```python
from build123d import *

# Parameters (mm, degrees)
F0_R     = 3
F0_R_2   = 6.530293
F1_DEPTH = 25


with BuildPart() as f1:
    # F0 (on Front) → F1 (new body)
    with BuildSketch(Plane.XZ):
        with BuildLine():
            ThreePointArc((24.831743, -2.895608), (24.9579, -1.450246), (25, 0))
            ThreePointArc((25, 0), (24.95158, 1.555208), (24.806506, 3.104392))
            ThreePointArc((24.806506, 3.104392), (24.498901, 4.980347), (24.04964, 6.827504))
            ThreePointArc((24.04964, 6.827504), (23.056544, 9.664149), (21.730224, 12.361123))
            ThreePointArc((21.730224, 12.361123), (20.728137, 13.976564), (19.606198, 15.51119))
            ThreePointArc((19.606198, 15.51119), (17.603159, 17.751867), (15.345712, 19.735986))
            ThreePointArc((15.345712, 19.735986), (13.801702, 20.844976), (12.177889, 21.833438))
            ThreePointArc((12.177889, 21.833438), (9.469853, 23.137024), (6.624954, 24.106223))
            ThreePointArc((6.624954, 24.106223), (4.774083, 24.539929), (2.895608, 24.831743))
            ThreePointArc((2.895608, 24.831743), (-0.105152, 24.999779), (-3.104392, 24.806506))
            ThreePointArc((-3.104392, 24.806506), (-4.980347, 24.498901), (-6.827504, 24.04964))
            ThreePointArc((-6.827504, 24.04964), (-9.664149, 23.056544), (-12.361123, 21.730224))
            ThreePointArc((-12.361123, 21.730224), (-13.976564, 20.728137), (-15.51119, 19.606198))
            ThreePointArc((-15.51119, 19.606198), (-17.751867, 17.603159), (-19.735986, 15.345712))
            ThreePointArc((-19.735986, 15.345712), (-20.844976, 13.801702), (-21.833438, 12.177889))
            ThreePointArc((-21.833438, 12.177889), (-23.137024, 9.469853), (-24.106223, 6.624954))
            ThreePointArc((-24.106223, 6.624954), (-24.539929, 4.774083), (-24.831743, 2.895608))
            ThreePointArc((-24.831743, 2.895608), (-24.999779, -0.105152), (-24.806506, -3.104392))
            ThreePointArc((-24.806506, -3.104392), (-24.498901, -4.980347), (-24.04964, -6.827504))
            ThreePointArc((-24.04964, -6.827504), (-23.056544, -9.664149), (-21.730224, -12.361123))
            ThreePointArc((-21.730224, -12.361123), (-20.728137, -13.976564), (-19.606198, -15.51119))
            ThreePointArc((-19.606198, -15.51119), (-17.603159, -17.751867), (-15.345712, -19.735986))
            ThreePointArc((-15.345712, -19.735986), (-13.801702, -20.844976), (-12.177889, -21.833438))
            ThreePointArc((-12.177889, -21.833438), (-9.469853, -23.137024), (-6.624954, -24.106223))
            ThreePointArc((-6.624954, -24.106223), (-4.774083, -24.539929), (-2.895608, -24.831743))
            ThreePointArc((-2.895608, -24.831743), (0.105152, -24.999779), (3.104392, -24.806506))
            ThreePointArc((3.104392, -24.806506), (4.980347, -24.498901), (6.827504, -24.04964))
            ThreePointArc((6.827504, -24.04964), (9.664149, -23.056544), (12.361123, -21.730224))
            ThreePointArc((12.361123, -21.730224), (13.976564, -20.728137), (15.51119, -19.606198))
            ThreePointArc((15.51119, -19.606198), (17.751867, -17.603159), (19.735986, -15.345712))
            ThreePointArc((19.735986, -15.345712), (20.844976, -13.801702), (21.833438, -12.177889))
            ThreePointArc((21.833438, -12.177889), (23.137024, -9.469853), (24.106223, -6.624954))
            ThreePointArc((24.106223, -6.624954), (24.539929, -4.774083), (24.831743, -2.895608))
        make_face()
        with Locations((-5.740251, -13.858193)):
            Circle(F0_R, mode=Mode.SUBTRACT)
        with Locations((10.606602, -10.606602)):
            Circle(F0_R, mode=Mode.SUBTRACT)
        with Locations((-15, 0)):
            Circle(F0_R, mode=Mode.SUBTRACT)
        Circle(F0_R_2, mode=Mode.SUBTRACT)
        with Locations((13.858193, 5.740251)):
            Circle(F0_R, mode=Mode.SUBTRACT)
        with Locations((0, 15)):
            Circle(F0_R, mode=Mode.SUBTRACT)
        with BuildLine():
            ThreePointArc((24.806506, 3.104392), (24.95158, 1.555208), (25, 0))
            ThreePointArc((25, 0), (24.9579, -1.450246), (24.831743, -2.895608))
            Line((24.831743, -2.895608), (30.030659, -1.999731))
            Line((30.030659, -1.999731), (29.965095, 1.999731))
            Line((29.965095, 1.999731), (24.806506, 3.104392))
        make_face()
        with BuildLine():
            ThreePointArc((21.730224, 12.361123), (23.056544, 9.664149), (24.04964, 6.827504))
            Line((24.04964, 6.827504), (28.509975, 9.644725))
            Line((28.509975, 9.644725), (26.918874, 13.314656))
            Line((26.918874, 13.314656), (21.730224, 12.361123))
        make_face()
        with BuildLine():
            Line((28.449402, -9.619635), (24.106223, -6.624954))
            ThreePointArc((24.106223, -6.624954), (23.137024, -9.469853), (21.833438, -12.177889))
            Line((21.833438, -12.177889), (26.979447, -13.339746))
            Line((26.979447, -13.339746), (28.449402, -9.619635))
        make_face()
        with BuildLine():
            ThreePointArc((15.345712, 19.735986), (17.603159, 17.751867), (19.606198, 15.51119))
            Line((19.606198, 15.51119), (22.648906, 19.820859))
            Line((22.648906, 19.820859), (19.774499, 22.602546))
            Line((19.774499, 22.602546), (15.345712, 19.735986))
        make_face()
        with BuildLine():
            Line((22.602546, -19.774499), (19.735986, -15.345712))
            ThreePointArc((19.735986, -15.345712), (17.751867, -17.603159), (15.51119, -19.606198))
            Line((15.51119, -19.606198), (19.820859, -22.648906))
            Line((19.820859, -22.648906), (22.602546, -19.774499))
        make_face()
        with BuildLine():
            ThreePointArc((6.624954, 24.106223), (9.469853, 23.137024), (12.177889, 21.833438))
            Line((12.177889, 21.833438), (13.339746, 26.979447))
            Line((13.339746, 26.979447), (9.619635, 28.449402))
            Line((9.619635, 28.449402), (6.624954, 24.106223))
        make_face()
        with BuildLine():
            Line((13.314656, -26.918874), (12.361123, -21.730224))
            ThreePointArc((12.361123, -21.730224), (9.664149, -23.056544), (6.827504, -24.04964))
            Line((6.827504, -24.04964), (9.644725, -28.509975))
            Line((9.644725, -28.509975), (13.314656, -26.918874))
        make_face()
        with BuildLine():
            ThreePointArc((-3.104392, 24.806506), (-0.105152, 24.999779), (2.895608, 24.831743))
            Line((2.895608, 24.831743), (1.999731, 30.030659))
            Line((1.999731, 30.030659), (-1.999731, 29.965095))
            Line((-1.999731, 29.965095), (-3.104392, 24.806506))
        make_face()
        with BuildLine():
            Line((1.999731, -29.965095), (3.104392, -24.806506))
            ThreePointArc((3.104392, -24.806506), (0.105152, -24.999779), (-2.895608, -24.831743))
            Line((-2.895608, -24.831743), (-1.999731, -30.030659))
            Line((-1.999731, -30.030659), (1.999731, -29.965095))
        make_face()
        with BuildLine():
            ThreePointArc((-12.361123, 21.730224), (-9.664149, 23.056544), (-6.827504, 24.04964))
            Line((-6.827504, 24.04964), (-9.644725, 28.509975))
            Line((-9.644725, 28.509975), (-13.314656, 26.918874))
            Line((-13.314656, 26.918874), (-12.361123, 21.730224))
        make_face()
        with BuildLine():
            Line((-9.619635, -28.449402), (-6.624954, -24.106223))
            ThreePointArc((-6.624954, -24.106223), (-9.469853, -23.137024), (-12.177889, -21.833438))
            Line((-12.177889, -21.833438), (-13.339746, -26.979447))
            Line((-13.339746, -26.979447), (-9.619635, -28.449402))
        make_face()
        with BuildLine():
            ThreePointArc((-19.735986, 15.345712), (-17.751867, 17.603159), (-15.51119, 19.606198))
            Line((-15.51119, 19.606198), (-19.820859, 22.648906))
            Line((-19.820859, 22.648906), (-22.602546, 19.774499))
            Line((-22.602546, 19.774499), (-19.735986, 15.345712))
        make_face()
        with BuildLine():
            Line((-19.774499, -22.602546), (-15.345712, -19.735986))
            ThreePointArc((-15.345712, -19.735986), (-17.603159, -17.751867), (-19.606198, -15.51119))
            Line((-19.606198, -15.51119), (-22.648906, -19.820859))
            Line((-22.648906, -19.820859), (-19.774499, -22.602546))
        make_face()
        with BuildLine():
            ThreePointArc((-24.106223, 6.624954), (-23.137024, 9.469853), (-21.833438, 12.177889))
            Line((-21.833438, 12.177889), (-26.979447, 13.339746))
            Line((-26.979447, 13.339746), (-28.449402, 9.619635))
            Line((-28.449402, 9.619635), (-24.106223, 6.624954))
        make_face()
        with BuildLine():
            Line((-26.918874, -13.314656), (-21.730224, -12.361123))
            ThreePointArc((-21.730224, -12.361123), (-23.056544, -9.664149), (-24.04964, -6.827504))
            Line((-24.04964, -6.827504), (-28.509975, -9.644725))
            Line((-28.509975, -9.644725), (-26.918874, -13.314656))
        make_face()
        with BuildLine():
            ThreePointArc((-24.806506, -3.104392), (-24.999779, -0.105152), (-24.831743, 2.895608))
            Line((-24.831743, 2.895608), (-30.030659, 1.999731))
            Line((-30.030659, 1.999731), (-29.965095, -1.999731))
            Line((-29.965095, -1.999731), (-24.806506, -3.104392))
        make_face()
    extrude(amount=F1_DEPTH)


solid = f1.part
```
Can you work these out from the model? Positions are in its coordinate system, mm. A direction names the side the tool comes from. Give positions to 0.01 mm unless a question says otherwise; leave off trailing zeros. Order: outer loops, then holes, each group sorted by start corner. A loop starts at its lowest first (then second) coordinate and runs counter-clockwise, first axis right, second up. Notation, with made-up numbers: (-25.5, 4) - (-8.5, 4) arc R11 cw to (-8.5, 15) - close; hole circle Ø11 at (29, 55). An arc over 180 degrees is marked (long way). Use a Markdown table: item, result. Add a question column.
Q1. If we section it at B-B on x = 0: Write out the boundary of the cut face in (y, z), plus the area to 3 significant figures.
Q2. If we section it at D-D on y = -14: Count the separate pieces of the cut face and the enclosed holes in it, plus the area to 3 significant figures.
Q3. If we mould it in two halves opening along X, with no side actions, what happens to faces 1 (the flat face through (0, 0, 7)), 2 (the flat face through (-8.216, -12.325, 26.249)), 3 (the flat face through (-27.704, -12.325, 11.506))? For each: released by +X, released by -X, zero draft, split by the parting line, or undercut.
Q4. I'm going to push flat-ended pins straight in: pin 1 (2 mm diameter, centred on y = -20.5, z = 15.5, fed in from -X); pin 2 (1.5 mm diameter, centred on x = -10.5, y = -21.5, fed in from +Z); pin 3 (10 mm diameter, centred on x = 8.5, y = -10, fed in from -Z). Where does each tip first touch, or does it pass through?
Q5. If we section it at A-A on x = -17: Write out the boundary of the cut face in (y, z), plus the area to 3 significant figures.
Q6. If we section it at C-C on z = 0: Write out the boundary of the cut face in (x, y).
Q7. Please list where these lines run through material, in increasing order: line 1 along Z through (x, y) = (22, -5); line 2 along X through (y, z) = (-4.75, -25.5); line 3 along X through (y, z) = (-16.5, -25).
Q8. On a 3-axis mill with a long thin cutter (end or side, diameter ignored), from which of +Z, -Z, +X, -X, +Y, -Y can I reach the whole of each face in a straight line? I mean faces 4 (the flat face through (-21.232, -12.325, -21.192)), 5 (the flat face through (2.454, -12.325, 27.395)), 6 (the flat face through (2.544, -12.325, -27.422)), 7 (the cylindrical face through (-20.83, -12.325, 13.824)). Say none if no direction works.
Answers follow:
| question | item | result |
|---|---|---|
| 1 | outline | (-25, -30) - (0, -30) - (0, -6.53) - (-25, -6.53) - close; (-25, 6.53) - (0, 6.53) - (0, 12) - (-25, 12) - close; (-25, 18) - (0, 18) - (0, 30) - (-25, 30) - close |
| 1 | area | 1,020 mm^2 |
| 2 | separate pieces | 1 |
| 2 | enclosed holes | 6 |
| 2 | area | 2,090 mm^2 |
| 3 | face 1 | zero draft |
| 3 | face 2 | undercut |
| 3 | face 3 | released by -X |
| 4 | pin 1 | stops at x = -20.48 |
| 4 | pin 2 | stops at z = 28.46 |
| 4 | pin 3 | stops at z = -28.51 |
| 5 | outline | (-25, -20.81) - (0, -20.81) - (0, -2.24) - (-25, -2.24) - close; (-25, 2.24) - (0, 2.24) - (0, 20.66) - (-25, 20.66) - close |
| 5 | area | 925 mm^2 |
| 6 | outline | (-30, -25) - (-18, -25) - (-18, 0) - (-30, 0) - close; (-12, -25) - (-6.53, -25) - (-6.53, 0) - (-12, 0) - close; (6.53, -25) - (30, -25) - (30, 0) - (6.53, 0) - close |
| 7 | line 1 | z = -20.4 to -18.84, -12.22 to 12.41, 18.9 to 20.45 |
| 7 | line 2 | x = -13.01 to -7.59, -2.78 to 2.96, 7.74 to 13.05 |
| 7 | line 3 | x = -12.89 to -7.24, -2.87 to 3.06, 7.43 to 12.96 |
| 8 | face 4 | -Z, -X, +Y, -Y |
| 8 | face 5 | +Z, +Y, -Y |
| 8 | face 6 | -Z, +Y, -Y |
| 8 | face 7 | +Y, -Y |
